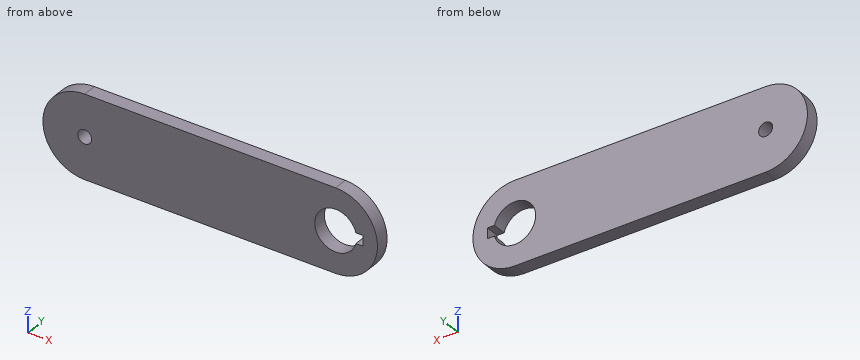
from build123d import *

# Parameters (mm, degrees)
BOSS_EXTRUDE1_DEPTH = 6.35
SKETCH3_R           = 3.175
CUT_EXTRUDE1_DEPTH  = 7.35


with BuildPart() as part:
    # Sketch1 → Boss-Extrude1 (new body)
    with BuildSketch(Plane(origin=(0, 0, 0), x_dir=(1, 0, 0), z_dir=(0, 1, 0))):
        with BuildLine():
            Line((0, 19.05), (114.3, 19.05))
            ThreePointArc((114.3, 19.05), (133.35, 0), (114.3, -19.05))
            Line((114.3, -19.05), (0, -19.05))
            ThreePointArc((0, -19.05), (-19.05, 0), (0, 19.05))
        make_face()
        with BuildLine():
            Line((123.522541593, -2.38125), (126.697541593, -2.38125))
            Line((126.697541593, -2.38125), (126.697541593, 2.38125))
            Line((126.697541593, 2.38125), (123.522541593, 2.38125))
            ThreePointArc((123.522541593, 2.38125), (104.775, 0), (123.522541593, -2.38125))
        make_face(mode=Mode.SUBTRACT)
    extrude(amount=BOSS_EXTRUDE1_DEPTH)

    # Sketch3 → Cut-Extrude1 (cut, through all)
    with BuildSketch(Plane(origin=(0, 6.35, 0), x_dir=(1, 0, 0), z_dir=(0, 1, 0))):
        Circle(SKETCH3_R)
    extrude(amount=-CUT_EXTRUDE1_DEPTH, mode=Mode.SUBTRACT)


solid = part.part
Geometry: final body of the model. Coordinates: model frame, mm. Coordinates: 2 decimals unless noted, no trailing zeros. Write each loop counter-clockwise with the first axis right and the second up, starting at its lowest first coordinate (ties: lowest second). Pieces come first, ordered by that corner, then holes. Notation, with made-up numbers: (20.5, 26) - (28.5, 26) arc R7 cw to (28.5, 34) - close; hole circle Ø4 at (29, -38.75). An arc over 180 degrees is marked (long way). Return JSON: item names as keys, results as strings.
Item 1: Line query: L1, parallel to X at y = 2.75, z = 0 (3 decimals); L2, parallel to X at y = 4.75, z = 2; L3, parallel to Z at x = 114.3, y = 2 (3 decimals). Output: solid intervals per line, ascending.
Completed:
{"L1": "x = -19.05 to -3.175, 3.175 to 104.775, 126.698 to 133.35", "L2": "x = -18.94 to -2.47, 2.47 to 104.99, 126.7 to 133.24", "L3": "z = -19.05 to -9.525, 9.525 to 19.05"}
Item 2: Section query C-C (x = -7). Output: boundary loops of the cut face in (y, z).
Completed:
{"outline": "(0, -17.72) - (6.35, -17.72) - (6.35, 17.72) - (0, 17.72) - close"}
Item 3: Pin query (flat end, axial travel): pin 1 Ø1.4 at (y, z) = (2, -0.5) entering from -X; pin 2 Ø2.5 at (x, y) = (125.5, 3) entering from +Z (3 decimals); pin 3 Ø2.5 at (x, y) = (124.5, 4) entering from -Z. Return the tip coordinate at first contact, or that it passes through.
Completed:
{"pin 1": "stops at x = -19.05", "pin 2": "stops at z = 16.245", "pin 3": "stops at z = -16.82"}
Item 4: Section query A-A (y = 4). Output: boundary loops of the cut face in (x, z) (3 decimals).
Completed:
{"outline": "(0, -19.05) - (114.3, -19.05) arc R19.05 ccw to (114.3, 19.05) - (0, 19.05) arc R19.05 ccw to start; hole circle Ø6.35 at (0, 0); hole (123.523, -2.381) - (126.698, -2.381) - (126.698, 2.381) - (123.523, 2.381) arc R9.525 ccw (long way) to start"}
Item 5: Section query B-B (z = 0). Output: boundary loops of the cut face in (x, y) (3 decimals), and give its area (3 significant figures).
Completed:
{"outline": "(-19.05, 0) - (-3.175, 0) - (-3.175, 6.35) - (-19.05, 6.35) - close; (3.175, 0) - (104.775, 0) - (104.775, 6.35) - (3.175, 6.35) - close; (126.698, 0) - (133.35, 0) - (133.35, 6.35) - (126.698, 6.35) - close", "area": "788 mm2"}
Item 6: Section query D-D (z = 16). Output: boundary loops of the cut face in (x, y), and give its area (3 significant figures).
Completed:
{"outline": "(-10.34, 0) - (124.64, 0) - (124.64, 6.35) - (-10.34, 6.35) - close", "area": "857 mm2"}
